Design review of the part built by this model. Coordinates are the model's own, in mm. A direction names the side the tool comes from. Round coordinates to 2 decimals unless told otherwise and drop trailing zeros. Loops run counter-clockwise (first coordinate to the right, second up) from the corner with the lowest first, then second, coordinate; pieces in that order, holes last. Notation, with made-up numbers: (1, 40.25) - (11, 40.25) arc R22 ccw to (11, 50.25) - close; hole circle Ø2 at (19.5, -31). An arc over 180 degrees is marked (long way). Return JSON: item names as keys, results as strings. Group by question number.
Autodesk Inventor part; units mm, degrees
ref_plane "YZ Plane" through (0, 0, 0) normal (1, 0, 0) x (0, 1, 0)
ref_plane "XZ Plane" through (0, 0, 0) normal (0, 1, 0) x (-1, 0, 0)
ref_plane "XY Plane" through (0, 0, 0) normal (0, 0, 1) x (1, 0, 0)
sketch "Sketch1" plane through (0, 0, 0) normal (0, 0, 1) x (1, 0, 0)
  line L0 (-31, -31) -> (31, -31)
  line L1 (31, -31) -> (31, 31)
  line L2 (31, 31) -> (-31, 31)
  line L3 (-31, 31) -> (-31, -31)
  line L4 (-31, -31) -> (31, 31) construction
  line L5 (31, -31) -> (-31, 31) construction
  line L6 (-33, 33) -> (33, 33)
  line L7 (33, 33) -> (33, -33)
  line L8 (33, -33) -> (-33, -33)
  line L9 (-33, -33) -> (-33, 33)
  point P0 (0, 0)
  dimension "d0" = 62
  dimension "d1" = 62
  dimension "d2" = 2
extrude "Extrusion1" add sketch "Sketch1" along normal blind 2 contours L3 L2 L1 L0 | L6 L7 L8 L9
extrude "Extrusion2" add sketch "Sketch1" against normal blind 12
sketch "Sketch2" plane through (-33, 33, 2) normal (0, 1, 0) x (1, 0, 0)
  line L0 (8, 3) -> (58, 3)
  line L1 (58, 3) -> (58, 0)
  line L2 (58, 0) -> (8, 0)
  line L3 (8, 0) -> (8, 3)
  line L4 (0, 14) -> (0, 0)
  line L5 (0, 14) -> (66, 14)
  point P0 (33, 2)
  dimension "d7" = 50
  dimension "d8" = 3
  dimension "d9" = 8
  dimension "d10" = 11
extrude "Extrusion3" add sketch "Sketch2" along normal blind 12
sketch "Sketch3" plane through (25, 33, -1) normal (0, 0, -1) x (-1, 0, 0)
  line L0 (50, 12) -> (0, 12)
  line L1 (50, 0) -> (50, 12)
  line L2 (0, 12) -> (50, 12)
  line L3 (50, 12) -> (50, 9)
  line L4 (50, 9) -> (0, 9)
  line L5 (0, 9) -> (0, 12)
  point P0 (25, -33)
  dimension "d13" = 3
extrude "Extrusion4" add sketch "Sketch3" along normal blind 60
sketch "Sketch7" plane through (-33, 45, 2) normal (0, 1, 0) x (1, 0, 0)
  circle A0 centre (32.875, 46) radius 6.45
  circle A1 centre (14.5, 46) radius 2.125
  circle A2 centre (51.25, 46) radius 2.125
  line L0 (14.5, 46) -> (32.875, 46)
  line L1 (32.875, 46) -> (51.25, 46)
  line L2 (51.6412, 48.0887) -> (37.1884, 50.7955)
  line L3 (51.25, 43.875) -> (37.6436, 41.6569)
  line L4 (14.5, 43.875) -> (28.1064, 41.6569)
  line L5 (14.5, 48.125) -> (28.5616, 50.7955)
  line L6 (58, 0) -> (58, 63)
  line L7 (8, 63) -> (58, 63)
  point P0 (33, 2)
  dimension "d34" = 12.9
  dimension "d35" = 4.25
  dimension "d36" = 4.25
  dimension "d37" = 41
  dimension "d38" = 9.15
  dimension "d39" = 6.75
  dimension "d40" = 17
extrude "Extrusion8" cut sketch "Sketch7" against normal blind 2.5
properties part number "pan_base_holder_third_v2"
Q1. Add section D-D, the plane z = -52. State the section outline as (x, y) points, plus the area to 3 significant figures.
Q2. Draft analysis for pull direction X (two halves, no side actions). For faces 1 (the flat face through (33, 0, -5)), 2 (the flat face through (0, 44, -61)), 3 (the flat face through (31, 0, -6)), state which applies: pulls with the +X half, pulls with the -X half, needs draft (parallel to the pull), parting line crosses it, or undercut.
Q3. For line 1 (Y direction, x = -7, z = -7); line 2 (X direction, y = 3.5, z = -11); line 3 (Z direction, x = -4.5, y = 19.5), list the stretches that pass through material, from the lowest coordinate up.
Q4. Insertion check: pin 1 Ø20 at (x, y) = (-15, 6.5) entering from -Z; pin 2 Ø4 at (x, z) = (0, -44) entering from +Y; pin 3 Ø13 at (y, z) = (39.5, -44.5) entering from -X. Each pin has a flat end and moves straight along its axis. Give the tip position at first contact, or say it passes through.
Q5. Add section B-B, the plane y = -22. State the section outline as (x, z) points, plus the area to 3 significant figures.
Q6. Tool access review of faces 4 (the flat face through (25, 43, -27)), 5 (the flat face through (0, -31, -6)), 6 (the flat face through (-11.57, 43.77, -47.44)): name each direction out of +Z, -Z, +X, -X, +Y, -Y from which nothing blocks a thin tool from reaching the whole face with its end or side.
Q7. Add section A-A, the plane z = -10. State the section outline as (x, y) points.
Evaluation:
{
 "1": {"outline": "(-25, 42) - (25, 42) - (25, 45) - (-25, 45) - close", "area": "150 mm²"},
 "2": {"face 1": "pulls with the +X half", "face 2": "needs draft", "face 3": "undercut"},
 "3": {"line 1": "-33 to -31, 31 to 33, 42 to 45", "line 2": "-33 to -31, 31 to 33", "line 3": "0 to 2"},
 "4": {"pin 1": "z = 0", "pin 2": "y = 42.5", "pin 3": "x = -25"},
 "5": {"outline": "(-33, -12) - (-31, -12) - (-31, 0) - (31, 0) - (31, -12) - (33, -12) - (33, 2) - (-33, 2) - close", "area": "180 mm²"},
 "6": {"face 4": "+Z, -Z, +X, +Y", "face 5": "-Z", "face 6": "+Y"},
 "7": {"outline": "(-33, -33) - (33, -33) - (33, 33) - (-33, 33) - close; (-25, 42) - (25, 42) - (25, 45) - (-25, 45) - close; hole (-31, -31) - (31, -31) - (31, 31) - (-31, 31) - close"}
}
